Verification items for the finished model (mm, model axes). Face numbers are marked on the shaded views. A direction names the side the tool comes from. Give positions to 0.01 mm unless a question says otherwise; leave off trailing zeros. Loops run counter-clockwise (first coordinate to the right, second up) from the corner with the lowest first, then second, coordinate; pieces in that order, holes last. Notation, with made-up numbers: M -31.75,-17.75 L -22.75,-17.75 A9 ccw -22.75,-11.75 Z; hole C 24.5,5.5 d8. An arc over 180 degrees is marked long. Answer in a Markdown table with one row per item.
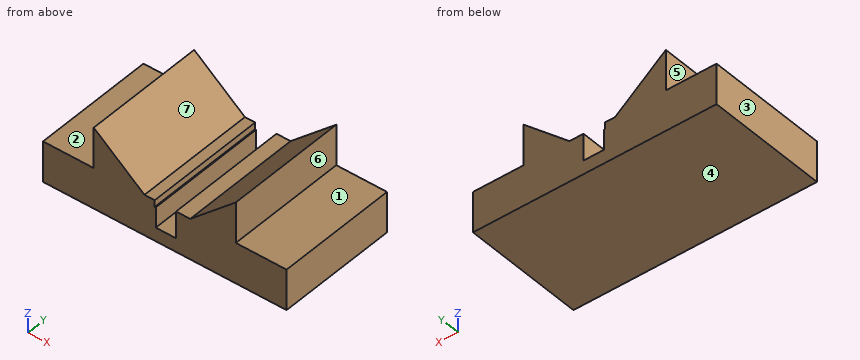
```python
from build123d import *

# Parameters (mm, degrees)
F0_W      = 152.4
F0_H      = 50.8
F1_DEPTH  = 76.2
F2_W      = 31.75
F2_H      = 25.4
F3_DEPTH  = 76.2
F4_W      = 31.75
F4_H      = 25.4
F5_DEPTH  = 76.2
F7_DEPTH  = 76.2
F9_DEPTH  = 76.2
F10_W     = 28.575
F10_H     = 25.4
F11_DEPTH = 76.2
F12_W     = 12.7
F12_H     = 12.7
F13_DEPTH = 101.6
F15_DEPTH = 101.6


with BuildPart() as f1:
    # F0 (on Front) → F1 (new body)
    with BuildSketch(Plane.XZ):
        with Locations((-0.381002, -49.234485)):
            Rectangle(F0_W, F0_H)
    extrude(amount=-F1_DEPTH)

    # F2 (on face) → F3 (cut)
    with BuildSketch(Plane.XZ):
        with Locations((-60.706002, -36.534485)):
            Rectangle(F2_W, F2_H)
    extrude(amount=-F3_DEPTH, mode=Mode.SUBTRACT)

    # F4 (on face) → F5 (cut)
    with BuildSketch(Plane.XZ):
        with Locations((59.943998, -36.534485)):
            Rectangle(F4_W, F4_H)
    extrude(amount=-F5_DEPTH, mode=Mode.SUBTRACT)

    # F6 (on face) → F7 (cut)
    with BuildSketch(Plane.XZ):
        Polygon((-13.081002, -23.834485), (-44.831002, -23.834485), (-13.081002, -49.234485), align=None)
    extrude(amount=-F7_DEPTH, mode=Mode.SUBTRACT)

    # F8 (on face) → F9 (cut)
    with BuildSketch(Plane.XZ):
        Polygon((44.068998, -23.834485), (15.493998, -23.834485), (15.493998, -49.234485), align=None)
    extrude(amount=-F9_DEPTH, mode=Mode.SUBTRACT)

    # F10 (on face) → F11 (cut)
    with BuildSketch(Plane.XZ):
        with Locations((1.206498, -36.534485)):
            Rectangle(F10_W, F10_H)
    extrude(amount=-F11_DEPTH, mode=Mode.SUBTRACT)

    # F12 (on face) → F13 (cut)
    with BuildSketch(Plane.XZ):
        with Locations((0.338951, -59.722185)):
            Rectangle(F12_W, F12_H)
    extrude(amount=-F13_DEPTH, mode=Mode.SUBTRACT)

    # F14 (on face) → F15 (cut)
    with BuildSketch(Plane.XZ):
        Polygon((6.688951, -49.234485), (-6.6675, -49.234485), (-6.6675, -53.372185), (-6.011049, -53.372185), (6.688951, -53.372185), align=None)
    extrude(amount=-F15_DEPTH, mode=Mode.SUBTRACT)


solid = f1.part
```
Item 1: Sectioned sample at C-C (z = -30). Record the cut outline in (x, y).
Reported:
| item | result |
|---|---|
| outline | M -44.83,0 L -37.12,0 L -37.12,76.2 L -44.83,76.2 Z; M 37.13,0 L 44.07,0 L 44.07,76.2 L 37.13,76.2 Z |
Item 2: Tool access check on the marked faces 1, 2 and 3. Record the directions out of +Z, -Z, +X, -X, +Y, -Y that give a thin tool (end or side, any length) a straight path to the whole face; none if there is none.
Reported:
| item | result |
|---|---|
| face 1 | +Z, +X, +Y, -Y |
| face 2 | +Z, -X, +Y, -Y |
| face 3 | +Z, -Z, -X, +Y, -Y |
Item 3: Sectioned sample at A-A (z = -64.5). Record the cut outline in (x, y).
Reported:
| item | result |
|---|---|
| outline | M -76.58,0 L -6.01,0 L -6.01,76.2 L -76.58,76.2 Z; M 6.69,0 L 75.82,0 L 75.82,76.2 L 6.69,76.2 Z |
Item 4: Go/stop test with flat-tipped pins: pin 1 (9.5 mm diameter, centred on x = -53, y = 19.5, fed in from +Z); pin 2 (2 mm diameter, centred on y = 28.5, z = -30, fed in from -X); pin 3 (2 mm diameter, centred on x = 29, z = -49.5, fed in from -Y); pin 4 (5 mm diameter, centred on y = 50, z = -29.5, fed in from +X). Record where each tip stops, or that it passes through.
Reported:
| item | result |
|---|---|
| pin 1 | stops at z = -49.23 |
| pin 2 | stops at x = -44.83 |
| pin 3 | stops at y = 0 |
| pin 4 | stops at x = 44.07 |
Item 5: Sectioned sample at B-B (y = 30). Record the cut outline in (x, z), and give its area (3 significant figures).
Reported:
| item | result |
|---|---|
| outline | M -76.58,-74.63 L 75.82,-74.63 L 75.82,-49.23 L 44.07,-49.23 L 44.07,-23.83 L 15.49,-49.23 L 6.69,-49.23 L 6.69,-66.07 L -6.01,-66.07 L -6.01,-53.37 L -6.67,-53.37 L -6.67,-49.23 L -13.08,-49.23 L -44.83,-23.83 L -44.83,-49.23 L -76.58,-49.23 Z |
| area | 4,420 mm^2 |
Item 6: Scan lines: L1, parallel to X at y = 31.5, z = -58.5; L2, parallel to X at y = 61, z = -53; L3, parallel to Z at x = 62, y = 32.5. Record each from-to range of solid material in increasing order. Write a range as [from, to].
Reported:
| item | result |
|---|---|
| L1 | x = [-76.58, -6.01], [6.69, 75.82] |
| L2 | x = [-76.58, -6.67], [6.69, 75.82] |
| L3 | z = [-74.63, -49.23] |
Item 7: Release check for a two-part mould opening along X. For the marked faces 4, 5, 6 and 7 record: released by +X, released by -X, zero draft, split by the parting line, or undercut.
Reported:
| item | result |
|---|---|
| face 4 | zero draft |
| face 5 | released by -X |
| face 6 | released by +X |
| face 7 | undercut |
Item 8: Sectioned sample at D-D (x = -60). Record the cut outline in (y, z).
Reported:
| item | result |
|---|---|
| outline | M 0,-74.63 L 76.2,-74.63 L 76.2,-49.23 L 0,-49.23 Z |
